The model under review builds one solid part; all positions refer to its coordinate system, in mm. Face numbers are marked on the shaded views. A direction names the side the tool comes from. Round coordinates to 2 decimals unless told otherwise and drop trailing zeros. Order: outer loops, then holes, each group sorted by start corner. A loop starts at its lowest first (then second) coordinate and runs counter-clockwise, first axis right, second up.
1) Consider section A-A (x = 12). Give the boundary of the cut face in (y, z).
2) Mouldability with a two-part tool opening along Z and no side actions: class the marked faces 4, 5 and 6 as pulls with the +Z half, pulls with the -Z half, needs draft (parallel to the pull), parting line crosses it, or undercut.
3) Consider section D-D (z = 24.5). Give the boundary of the cut face in (x, y), then the cut area to 3 significant figures.
4) Consider section C-C (z = 10). Give the boundary of the cut face in (x, y).
5) To check wall thickness, follow L1, parallel to Y at x = 15, z = 3; L2, parallel to Z at x = 23.5, y = 26; L3, parallel to Y at x = 28.5, z = 14. State the ranges of each line that lie inside material, in increasing order.
6) Consider section B-B (y = 6). Give the boundary of the cut face in (x, z), then the cut area to 3 significant figures.
7) Clearance check with flat-ended pins moving along their axes: P1, Ø1.5, axis at x = 14, z = 2.5, coming from the +Y side; P2, Ø3.5, axis at x = 28, z = 42, coming from the -Y side; P3, Ø2.5, axis at x = 12, z = 3.5, coming from the -Y side; P4, Ø2.5, axis at y = 25.34, z = 10, coming from the +X side. State where each tip first meets the part, or that it passes through.
8) Machinability: for the marked faces 1, 2 and 3, which of the approach directions +Z, -Z, +X, -X, +Y, -Y give a long, thin tool a straight path to every point of the face, cutting with its end or side? Answer none if there is none.
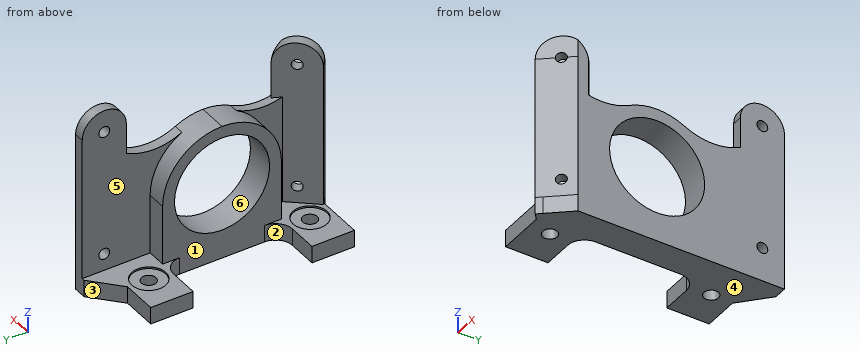
from build123d import *

# Parameters (mm, degrees)
EXTRUDE_2_DEPTH                = 5
SKETCH_4_W                     = 8.676470589
SKETCH_4_H                     = 35
SKETCH_4_W_2                   = 8.676470588
EXTRUDE_15_DEPTH               = 35
CUT_EXTRUDE_1_DEPTH            = 45
SKETCH_6_R                     = 14
CUT_EXTRUDE_2_DEPTH            = 45
FILLET_1_R                     = 5
SKETCH_7_R                     = 15
SKETCH_7_R_2                   = 13
EXTRUDE_16_DEPTH               = 1
SPLIT_BODIES_1_SURFACE_1_BACK  = 86
SPLIT_BODIES_1_SURFACE_1_DEPTH = 172
SPLIT_BODIES_1_SURFACE_2_BACK  = 86
SPLIT_BODIES_1_SURFACE_2_DEPTH = 172
HOLE_WIZARD_1_D                = 4.3
HOLE_WIZARD_1_DEPTH            = 5
HOLE_WIZARD_1_CBORE_D          = 10
HOLE_WIZARD_1_CBORE_DEPTH      = 0.5
HOLE_WIZARD_1_TIP              = 1.291850331
SKETCH_17_W                    = 3
SKETCH_17_H                    = 13
EXTRUDE_20_DEPTH               = 42
EXTRUDE_21_DEPTH               = 3
SKETCH_19_R                    = 1.6
CUT_EXTRUDE_3_DEPTH            = 3
EXTRUDE_START                  = -3
EXTRUDE_25_DEPTH               = 3
EXTRUDE_22_DEPTH               = 5
EXTRUDE_26_DEPTH               = 42
EXTRUDE_START_2                = -2.6
EXTRUDE_27_DEPTH               = 2.6
CUT_EXTRUDE_5_DEPTH            = 22.6
EXTRUDE_29_REACH               = 85.035
SKETCH_42_R                    = 1.5
CUT_EXTRUDE_6_DEPTH            = 84.034846606
CUT_EXTRUDE_7_DEPTH            = 8.6
EXTRUDE_31_DEPTH               = 5


with BuildPart() as part:
    # 草图2 → 凸台-拉伸2 (new body)
    with BuildSketch(Plane.XY):
        Polygon((7.726423565, 24.338235294), (-14.773576435, 24.338235294), (-14.773576435, -35.661764706), (7.726423565, -35.661764706), (7.726423565, -23.161764706), (-6.097105846, -23.161764706), (-6.097105846, 11.838235294), (7.726423565, 11.838235294), align=None)
        Polygon((30.226423565, 24.338235294), (7.726423565, 24.338235294), (7.726423565, 11.838235294), (21.549952977, 11.838235294), (21.549952977, -23.161764706), (7.726423565, -23.161764706), (7.726423565, -35.661764706), (30.226423565, -35.661764706), align=None)
    extrude(amount=EXTRUDE_2_DEPTH)

    # 草图4 → 凸台-拉伸15 (add)
    with BuildSketch(Plane.XY.offset(5)):
        with Locations((-10.435341141, -5.661764706)):
            Rectangle(SKETCH_4_W, SKETCH_4_H)
        with Locations((25.888188271, -5.661764706)):
            Rectangle(SKETCH_4_W_2, SKETCH_4_H)
    extrude(amount=EXTRUDE_15_DEPTH)

    # 草图5 → 切除-拉伸1 (cut)
    with BuildSketch(Plane.ZY.offset(14.773576435)):
        with BuildLine():
            Line((40, -23.161764706), (40, -5.661764706))
            ThreePointArc((40, -5.661764706), (34.874368671, -18.036133377), (22.5, -23.161764706))
            Line((22.5, -23.161764706), (40, -23.161764706))
        make_face()
        with BuildLine():
            ThreePointArc((22.5, 11.838235294), (34.874368671, 6.712603965), (40, -5.661764706))
            Line((40, -5.661764706), (40, 11.838235294))
            Line((40, 11.838235294), (22.5, 11.838235294))
        make_face()
    extrude(amount=-CUT_EXTRUDE_1_DEPTH, mode=Mode.SUBTRACT)

    # 草图6 → 切除-拉伸2 (cut)
    with BuildSketch(Plane.ZY.offset(14.773576435)):
        with Locations((22.5, -5.661764706)):
            Circle(SKETCH_6_R)
    extrude(amount=-CUT_EXTRUDE_2_DEPTH, mode=Mode.SUBTRACT)

    # 圆角1
    fillet_1_edges = [part.edges().sort_by_distance(p)[0] for p in [
        (-6.097105846, 11.838235294, 2.5),
        (-6.097105846, -23.161764706, 2.5),
        (21.549952977, -23.161764706, 2.5),
        (21.549952977, 11.838235294, 2.5),
    ]]
    fillet(fillet_1_edges, radius=FILLET_1_R)

    # 草图7 → 凸台-拉伸16 (add)
    with BuildSketch(Plane(origin=(-6.097105846, 0, 0), x_dir=(0, 0, -1), z_dir=(1, 0, 0))):
        with Locations((-22.5, -5.661764706)):
            Circle(SKETCH_7_R)
        with Locations((-22.5, -5.661764706)):
            Circle(SKETCH_7_R_2, mode=Mode.SUBTRACT)
    extrude(amount=-EXTRUDE_16_DEPTH)


with BuildPart() as body_2:
    # Split Bodies 1: the piece behind the surface
    add(part.part)
    # Split Bodies 1 surface: a surface, the sketch's curves swept straight by 172 mm
    with BuildLine(Plane.XY.offset(5).offset(-SPLIT_BODIES_1_SURFACE_1_BACK), mode=Mode.PRIVATE) as split_bodies_1_surface_1_path:
        Line((7.726423565, 24.338235294), (7.726423565, -35.661764706))
    split_bodies_1_surface_1 = Shell.extrude(split_bodies_1_surface_1_path.wire(), (0 * SPLIT_BODIES_1_SURFACE_1_DEPTH, 0 * SPLIT_BODIES_1_SURFACE_1_DEPTH, 1 * SPLIT_BODIES_1_SURFACE_1_DEPTH))
    split(bisect_by=split_bodies_1_surface_1, keep=Keep.BOTTOM)


with BuildPart() as part_1:
    add(part.part)

    # Split Bodies 1: split by a surface, the side it looks to stays
    # Split Bodies 1 surface: a surface, the sketch's curves swept straight by 172 mm
    with BuildLine(Plane.XY.offset(5).offset(-SPLIT_BODIES_1_SURFACE_2_BACK), mode=Mode.PRIVATE) as split_bodies_1_surface_2_path:
        Line((7.726423565, 24.338235294), (7.726423565, -35.661764706))
    split_bodies_1_surface_2 = Shell.extrude(split_bodies_1_surface_2_path.wire(), (0 * SPLIT_BODIES_1_SURFACE_2_DEPTH, 0 * SPLIT_BODIES_1_SURFACE_2_DEPTH, 1 * SPLIT_BODIES_1_SURFACE_2_DEPTH))
    split(bisect_by=split_bodies_1_surface_2, keep=Keep.TOP)

    # 打孔尺寸(%根据六角头螺)栓 全螺纹的类型1
    with Locations(Plane(origin=(18.226423565, 18.088235294, 5), x_dir=(1, 0, 0), z_dir=(0, 0, 1))):
        with Locations((0, 0), (0, -47.5)):
            CounterBoreHole(HOLE_WIZARD_1_D / 2, HOLE_WIZARD_1_CBORE_D / 2, HOLE_WIZARD_1_CBORE_DEPTH, depth=HOLE_WIZARD_1_DEPTH)
            with Locations((0, 0, -(HOLE_WIZARD_1_DEPTH + HOLE_WIZARD_1_TIP / 2))):  # 118° drill point
                Cone(0, HOLE_WIZARD_1_D / 2, HOLE_WIZARD_1_TIP, mode=Mode.SUBTRACT)

    # 草图17 → 凸台-拉伸20 (add)
    with BuildSketch(Plane.XY.offset(5)):
        with Locations((28.726423565, 25.338235294)):
            Rectangle(SKETCH_17_W, SKETCH_17_H)
    extrude(amount=EXTRUDE_20_DEPTH)

    # 草图18 → 凸台-拉伸21 (add)
    with BuildSketch(Plane(origin=(30.226423565, 0, 0), x_dir=(0, 0, -1), z_dir=(1, 0, 0))):
        with BuildLine():
            Line((-47, 18.838235294), (-47, 31.838235294))
            ThreePointArc((-47, 31.838235294), (-53.5, 25.338235294), (-47, 18.838235294))
        make_face()
    extrude(amount=-EXTRUDE_21_DEPTH)

    # 草图19 → 切除-拉伸3 (cut)
    with BuildSketch(Plane(origin=(30.226423565, 0, 0), x_dir=(0, 0, -1), z_dir=(1, 0, 0))):
        with Locations((-47, 25.338235294)):
            Circle(SKETCH_19_R)
        with Locations((-10, 25.338235294)):
            Circle(SKETCH_19_R)
    extrude(amount=-CUT_EXTRUDE_3_DEPTH, mode=Mode.SUBTRACT)

    # 草图24 → 凸台-拉伸25 (add)
    with BuildSketch(Plane(origin=(30.226423565, 0, 0), x_dir=(0, 0, -1), z_dir=(1, 0, 0)).offset(EXTRUDE_START)):
        with BuildLine():
            Line((-5, 18.838235294), (-38, 18.838235294))
            ThreePointArc((-38, 18.838235294), (-35.984258471, 10.650254496), (-38, 2.462273699))
            ThreePointArc((-38, 2.462273699), (-31.557574949, 9.311890026), (-22.5, 11.838235294))
            Line((-22.5, 11.838235294), (-5, 11.838235294))
            Line((-5, 11.838235294), (-5, 18.838235294))
        make_face()
    extrude(amount=EXTRUDE_25_DEPTH)

    # 草图21 → 凸台-拉伸22 (add)
    with BuildSketch(Plane.XY.offset(5)):
        Polygon((18.226423565, 24.338235294), (30.226423565, 24.338235294), (30.226423565, 31.838235294), (26.408241747, 31.838235294), align=None)
    extrude(amount=-EXTRUDE_22_DEPTH)

    # 草图34 → 凸台-拉伸26 (add)
    with BuildSketch(Plane.XY.offset(5)):
        Polygon((21.07205131, -35.191979637), (23.370184639, -37.120342466), (30.226423565, -28.949395095), (30.226423565, -25.903115259), (29.428290236, -25.233401877), align=None)
    extrude(amount=EXTRUDE_26_DEPTH)

    # 草图37 → 凸台-拉伸27 (add)
    with BuildSketch(Plane(origin=(30.226423565, 0, 0), x_dir=(0, 0, -1), z_dir=(1, 0, 0)).offset(EXTRUDE_START_2)):
        with BuildLine():
            Line((-37.42228501, -28.949395095), (-5, -28.949395095))
            Line((-5, -28.949395095), (-5, -23.161764706))
            Line((-5, -23.161764706), (-22.5, -23.161764706))
            ThreePointArc((-22.5, -23.161764706), (-31.557574949, -20.635419438), (-38, -13.785803111))
            ThreePointArc((-38, -13.785803111), (-35.997045319, -21.302294019), (-37.42228501, -28.949395095))
        make_face()
    extrude(amount=EXTRUDE_27_DEPTH)

    # 草图38 → 切除-拉伸5 (cut)
    with BuildSketch(Plane.XY.offset(5)):
        Polygon((30.226423565, -35.661764706), (30.226423565, -28.949395095), (24.5940767, -35.661764706), align=None)
    extrude(amount=-CUT_EXTRUDE_5_DEPTH, mode=Mode.SUBTRACT)

    # 凸台-拉伸29: up to this face of the body (flat: up to its plane)
    extrude_29_end = Plane(part_1.part.faces().sort_by_distance((24.617542998, -30.966627181, 27.010629393))[0])
    # 草图41 → 凸台-拉伸29 (add, up to the picked face)
    with BuildSketch(Plane(origin=(31.992387835, -26.844800832, 0), x_dir=(0, 0, -1), z_dir=(0.7660444431189818, -0.6427876096865348, 0)), mode=Mode.PRIVATE) as extrude_29_sk1:
        with BuildLine():
            Line((-47, -13.413766951), (-47, -0.413766951))
            ThreePointArc((-47, -0.413766951), (-53.5, -6.913766951), (-47, -13.413766951))
        make_face()
    extrude_29_tool1 = split(extrude(extrude_29_sk1.sketch, amount=-EXTRUDE_29_REACH, mode=Mode.PRIVATE), bisect_by=extrude_29_end, keep=Keep.BOTH, mode=Mode.PRIVATE)
    add(extrude_29_tool1.solids().sort_by(Axis((27.548304, -32.141054, 49.758686), (-0.7660444431189818, 0.6427876096865348, 0)))[0])

    # 草图42 → 切除-拉伸6 (cut, through all)
    with BuildSketch(Plane(origin=(31.992387835, -26.844800832, 0), x_dir=(0, 0, -1), z_dir=(0.7660444431189818, -0.6427876096865348, 0))):
        with Locations(Location((-47, -6.913766951, 0), (0, 0, 90))):
            Circle(SKETCH_42_R)
        with Locations(Location((-10, -6.913766951, 0), (0, 0, 90))):
            Circle(SKETCH_42_R)
    extrude(amount=-CUT_EXTRUDE_6_DEPTH, mode=Mode.SUBTRACT)

    # 草图44 → 切除-拉伸7 (cut)
    with BuildSketch(Plane(origin=(0, 0, 47), x_dir=(-1, 0, 0), z_dir=(0, 0, -1))):
        Polygon((-31.726423565, -27.161764706), (-30.226423565, -28.949395095), (-30.226423565, -25.903115259), align=None)
    extrude(amount=-CUT_EXTRUDE_7_DEPTH, mode=Mode.SUBTRACT)

    # 草图39 → 凸台-拉伸31 (add)
    with BuildSketch(Plane.XY.offset(5)):
        Polygon((24.5940767, -35.661764706), (21.631919353, -35.661764706), (23.370184639, -37.120342466), align=None)
    extrude(amount=-EXTRUDE_31_DEPTH)


solid = part_1.part
Answer below:
1. outline: (-35.66, 0) - (-23.16, 0) - (-23.16, 5) - (-35.66, 5) - close; (11.84, 0) - (24.34, 0) - (24.34, 5) - (11.84, 5) - close
2. face 4: pulls with the -Z half
2. face 5: needs draft
2. face 6: undercut
3. outline: (21.07, -35.19) - (23.37, -37.12) - (30.23, -28.95) - (30.23, -19.52) - (21.55, -19.52) - (21.55, -23.05) - (27.63, -23.05) - (27.63, -27.38) - close; (21.55, 8.19) - (30.23, 8.19) - (30.23, 31.84) - (27.23, 31.84) - (27.23, 11.72) - (21.55, 11.72) - close
3. area: 166 mm2
4. outline: (21.07, -35.19) - (23.37, -37.12) - (26.58, -33.29) - (24.29, -31.36) - close; (21.55, -23.16) - (27.63, -23.16) - (27.63, -27.38) - (26.21, -29.06) - (28.51, -30.99) - (30.23, -28.95) - (30.23, -11.97) - (21.55, -11.97) - close; (21.55, 0.64) - (30.23, 0.64) - (30.23, 23.74) - (27.23, 23.74) - (27.23, 11.84) - (21.55, 11.84) - close; (27.23, 26.94) - (30.23, 26.94) - (30.23, 31.84) - (27.23, 31.84) - close
5. L1: y = -35.66 to -23.16, 11.84 to 24.34
5. L2: z = 0 to 5
5. L3: y = -31.01 to -16.79, 5.46 to 31.84
6. outline: (21.55, 0) - (30.23, 0) - (30.23, 14.75) - (21.55, 14.75) - close; (21.55, 30.25) - (30.23, 30.25) - (30.23, 36.61) - (27.23, 36.61) - (27.23, 35.55) - (21.55, 35.55) - close
6. area: 177 mm2
7. P1: stops at y = 24.34
7. P2: stops at y = -33.69
7. P3: stops at y = -35.66
7. P4: passes through
8. face 1: +Z, -X
8. face 2: +Z, -Z, -X
8. face 3: +Z, -Z, -X, +Y
